The drawing under review shows one solid part. Ordinate dimensions are in mm from its lowest x, y, z. Round coordinates to 2 decimals unless told otherwise and drop trailing zeros. Order: outer loops, then holes, each group sorted by start corner. A loop starts at its lowest first (then second) coordinate and runs counter-clockwise, first axis right, second up. Notation, with made-up numbers: M -29,-12 L -9,-12 A24 cw -9,13 Z; hole C 86.5,-10 d3. An arc over 180 degrees is marked long. Answer in a Markdown table with one row per item. Add a question column.
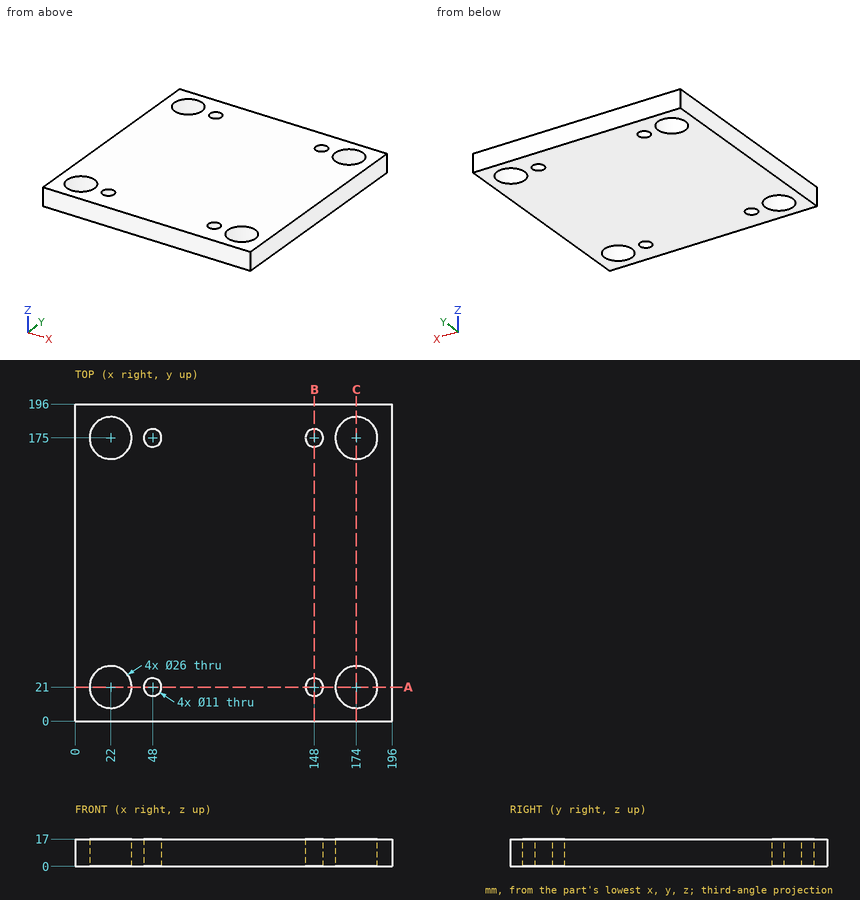
1. Consider section B-B on x = 148. Write out the cut boundary in (y, z), plus the area to 3 significant figures.
2. Consider section A-A on y = 21. Write out the cut boundary in (x, z), plus the area to 3 significant figures.
3. Clearance check with flat-ended pins moving along their axes: pin 1 Ø12.5 at (x, y) = (148, 175) entering from +Z; pin 2 Ø10 at (x, y) = (48, 21) entering from -Z. State where each tip first meets the part, or that it passes through.
4. To check wall thickness, follow probe 1 along Y at (x, z) = (174, 6.75); probe 2 along X at (y, z) = (21, 13); probe 3 along Y at (x, z) = (29.5, 5). State the ranges of each line that lie inside material, in increasing order. Write a range as [from, to].
5. Consider section C-C on x = 174. Write out the cut boundary in (y, z).
Solved:
| question | item | result |
|---|---|---|
| 1 | outline | M 0,0 L 15.5,0 L 15.5,17 L 0,17 Z; M 26.5,0 L 169.5,0 L 169.5,17 L 26.5,17 Z; M 180.5,0 L 196,0 L 196,17 L 180.5,17 Z |
| 1 | area | 2,960 mm^2 |
| 2 | outline | M 0,0 L 9,0 L 9,17 L 0,17 Z; M 35,0 L 42.5,0 L 42.5,17 L 35,17 Z; M 53.5,0 L 142.5,0 L 142.5,17 L 53.5,17 Z; M 153.5,0 L 161,0 L 161,17 L 153.5,17 Z; M 187,0 L 196,0 L 196,17 L 187,17 Z |
| 2 | area | 2,070 mm^2 |
| 3 | pin 1 | stops at z = 17 |
| 3 | pin 2 | passes through |
| 4 | probe 1 | y = [0, 8], [34, 162], [188, 196] |
| 4 | probe 2 | x = [0, 9], [35, 42.5], [53.5, 142.5], [153.5, 161], [187, 196] |
| 4 | probe 3 | y = [0, 10.38], [31.62, 164.38], [185.62, 196] |
| 5 | outline | M 0,0 L 8,0 L 8,17 L 0,17 Z; M 34,0 L 162,0 L 162,17 L 34,17 Z; M 188,0 L 196,0 L 196,17 L 188,17 Z |
